Design review of the part built by this model. Coordinates are the model's own, in mm. A direction names the side the tool comes from. Round coordinates to 2 decimals unless told otherwise and drop trailing zeros. Order: outer loops, then holes, each group sorted by start corner. A loop starts at its lowest first (then second) coordinate and runs counter-clockwise, first axis right, second up. Notation, with made-up numbers: (50.5, 75) - (107.5, 75) arc R26 cw to (107.5, 103) - close; hole circle Ø7 at (47, -4.75). An arc over 180 degrees is marked (long way). Write item = value, one per line.
from build123d import *

# Parameters (mm, degrees)
SKETCH1_R           = 1.25
BOSS_EXTRUDE1_DEPTH = 18
SKETCH4_R           = 2.25
BOSS_EXTRUDE2_DEPTH = 1.5
CUT_EXTRUDE1_DEPTH  = 0.5


with BuildPart() as part:
    # Sketch1 → Boss-Extrude1 (new body)
    with BuildSketch(Plane(origin=(0, 0, 0), x_dir=(1, 0, 0), z_dir=(0, 1, 0))):
        Circle(SKETCH1_R)
    extrude(amount=BOSS_EXTRUDE1_DEPTH)

    # Sketch4 → Boss-Extrude2 (add)
    with BuildSketch(Plane(origin=(0, 18, 0), x_dir=(1, 0, 0), z_dir=(0, 1, 0))):
        Circle(SKETCH4_R)
    extrude(amount=BOSS_EXTRUDE2_DEPTH)

    # Sketch5 → Cut-Extrude1 (cut)
    with BuildSketch(Plane(origin=(0, 19.5, 0), x_dir=(1, 0, 0), z_dir=(0, 1, 0))):
        Polygon((1.25, 0), (0.625, 1.082531755), (-0.625, 1.082531755), (-1.25, 0), (-0.625, -1.082531755), (0.625, -1.082531755), align=None)
    extrude(amount=-CUT_EXTRUDE1_DEPTH, mode=Mode.SUBTRACT)


solid = part.part
1) For faces 4 (the flat face through (0, 0, 0)), 5 (the flat face through (1, 18, 1)), list the 3-axis set-ups (+Z, -Z, +X, -X, +Y, -Y) from which the entire face can be reached by the end or side of a thin tool; tool diameter is ignored.
Findings:
face_4 = +Z, -Z, +X, -X, -Y
face_5 = -Y
2) The part is to be moulded in two halves that separate along Z. For faces 1 (the cylindrical face through (-0.29, 18.74, -2.23)), 2 (the flat face through (0, 19, 0)), 3 (the flat face through (1, 19.5, -1)), say which applies: released by +Z, released by -Z, zero draft, split by the parting line, or undercut.
Findings:
face_1 = split by the parting line
face_2 = undercut
face_3 = zero draft
3) We need section A-A on x = 0. Write out the cut boundary in (y, z), and give its area (3 significant figures).
Findings:
outline = (0, -1.25) - (18, -1.25) - (18, -2.25) - (19.5, -2.25) - (19.5, -1.08) - (19, -1.08) - (19, 1.08) - (19.5, 1.08) - (19.5, 2.25) - (18, 2.25) - (18, 1.25) - (0, 1.25) - close
area = 50.7 mm^2
4) We need section C-C on y = 12.5. Write out the cut boundary in (x, z).
Findings:
outline = circle Ø2.5 at (0, 0)
5) Clearance check with flat-ended pins moving along their axes: pin 1 Ø2 at (y, z) = (16.5, 0) entering from -X; pin 2 Ø1 at (x, y) = (-0.5, 9) entering from +Z; pin 3 Ø1.5 at (x, y) = (1.5, 3) entering from -Z; pin 4 Ø2 at (x, z) = (-1.5, 1) entering from -Y. State where each tip first meets the part, or that it passes through.
Findings:
pin_1 = -1.25
pin_2 = 1.25
pin_3 = -1
pin_4 = 0
6) We need section B-B on z = 0.55. Write out the cut boundary in (x, y).
Findings:
outline = (-2.18, 18) - (-1.12, 18) - (-1.12, 0) - (1.12, 0) - (1.12, 18) - (2.18, 18) - (2.18, 19.5) - (0.93, 19.5) - (0.93, 19) - (-0.93, 19) - (-0.93, 19.5) - (-2.18, 19.5) - close
7) To check wall thickness, follow L1, parallel to Y at x = -0.1, z = 1.5; L2, parallel to Y at x = -0.15, z = -0.65; L3, parallel to X at y = 14.25, z = 0. State the ranges of each line that lie inside material, in increasing order. Write a range as from..to.
Findings:
L1 = 18..19.5
L2 = 0..19
L3 = -1.25..1.25
8) We need section D-D on x = 1.7. Write out the cut boundary in (y, z), and give its area (3 significant figures).
Findings:
outline = (18, -1.47) - (19.5, -1.47) - (19.5, 1.47) - (18, 1.47) - close
area = 4.42 mm^2
